Check sheet for the modelled part. Datum: model origin and axes. Units: mm. A direction names the side the tool comes from. Give positions to 0.01 mm unless a question says otherwise; leave off trailing zeros. Loops run counter-clockwise (first coordinate to the right, second up) from the corner with the lowest first, then second, coordinate; pieces in that order, holes last. Notation, with made-up numbers: M -19,-38 L 4,-38 A24 ccw 4,-20 Z; hole C 31,63 d9. An arc over 180 degrees is marked long. Write each question's results on one line, items separated by ' | '. Start each with the question number.
1. Material ranges on line 1 along X through (y, z) = (9.1, 15); line 2 along X through (y, z) = (7.45, 15); line 3 along Z through (x, y) = (-14.5, -0.5), recorded low to high.
2. Draft check along X on faces 6 (the flat face through (4, 11, -25)), 7 (the flat face through (-12.25, 5, -50)), 8 (the flat face through (16, 8, 19)), 9 (the flat face through (20, 4, -26)). Enter one of: pulls with the +X half, pulls with the -X half, needs draft (parallel to the pull), parting line crosses it, or undercut.
3. Sectioned sample at A-A on y = -3.5. Record the cut outline in (x, z).
4. Tool access check on faces 1 (the flat face through (3, 1, -25)), 2 (the flat face through (9, 11, -35.75)), 3 (the flat face through (-12, 8, -65)), 4 (the flat face through (-15, 8, -63)), 5 (the flat face through (7, 14, -39)). Record the directions out of +Z, -Z, +X, -X, +Y, -Y that give a thin tool (end or side, any length) a straight path to the whole face; none if there is none.
5. Go/stop test with flat-tipped pins: pin 1 (1.5 mm diameter, centred on y = 8, z = -26, fed in from -X); pin 2 (12 mm diameter, centred on x = -2.5, y = 6, fed in from -Z); pin 3 (1.5 mm diameter, centred on x = 0.5, z = -25.5, fed in from -Y). Record where each tip stops, or that it passes through.
6. Sectioned sample at C-C on z = -65. Record the cut outline in (x, y).
7. Sectioned sample at B-B on x = -16. Give the number of separate pieces and of enclosed holes in the cut face, and give its area (3 significant figures).
```python
from build123d import *

# Parameters (mm, degrees)
SKETCH1_W                  = 40
SKETCH1_H                  = 22
BOSS_EXTRUDE1_DEPTH        = 11
SKETCH2_W                  = 40
SKETCH2_H                  = 22
SKETCH2_R                  = 7.843750423
BOSS_EXTRUDE2_DEPTH        = 5
SKETCH3_W                  = 24.5
SKETCH3_H                  = 15.5
CUT_EXTRUDE1_DEPTH         = 7.75
FILLET1_R                  = 7.75
SKETCH4_R                  = 5
CUT_EXTRUDE2_DEPTH         = 36.805900352
SKETCH5_W                  = 8
SKETCH5_H                  = 8
SKETCH5_R                  = 1.905800151
BOSS_EXTRUDE3_DEPTH        = 6
CUT_EXTRUDE3_START         = -3
SKETCH6_R                  = 3
SKETCH6_R_2                = 1.905800151
CUT_EXTRUDE3_DEPTH         = 3
SKETCH7_W                  = 16
SKETCH7_H                  = 16.5
BOSS_EXTRUDE5_DEPTH        = 28
MIRROR14_COPY_1_SKETCH_W   = 8
MIRROR14_COPY_1_SKETCH_H   = 8
MIRROR14_COPY_1_SKETCH_R   = 1.905800151
MIRROR14_COPY_1_DEPTH      = 6
MIRROR14_START             = -3
MIRROR14_COPY_2_SKETCH_R   = 3
MIRROR14_COPY_2_SKETCH_R_2 = 1.905800151
MIRROR14_COPY_2_DEPTH      = 3
FILLET1_OF_MIRROR14_R      = 7.75
SKETCH9_W                  = 28
SKETCH9_H                  = 3
BOSS_EXTRUDE6_DEPTH        = 18
CUT_EXTRUDE4_DEPTH         = 10
CUT_EXTRUDE5_DEPTH         = 73.919476136
CUT_EXTRUDE5_DEPTH_BACK    = 73.919476136
SKETCH11_R                 = 1.75
CUT_EXTRUDE6_DEPTH         = 76.121568141
CUT_EXTRUDE6_DEPTH_BACK    = 76.121568141
SKETCH12_R                 = 1.75
CUT_EXTRUDE9_DEPTH         = 12
CUT_EXTRUDE11_START        = -10
SKETCH16_R                 = 4
SKETCH16_R_2               = 1.75
SKETCH16_W                 = 10
SKETCH16_H                 = 6.5
CUT_EXTRUDE11_DEPTH        = 10
FILLET2_R                  = 2
CUT_EXTRUDE12_START        = -3
SKETCH17_R                 = 1.75
CUT_EXTRUDE12_DEPTH        = 3


# Some blends are built 0.0001 mm under size
with BuildPart() as part:
    # Sketch1 → Boss-Extrude1 (new body)
    with BuildSketch(Plane(origin=(0, 0, 0), x_dir=(1, 0, 0), z_dir=(0, 1, 0))):
        Rectangle(SKETCH1_W, SKETCH1_H)
    boss_extrude1 = extrude(amount=BOSS_EXTRUDE1_DEPTH)

    # Sketch2 → Boss-Extrude2 (add)
    with BuildSketch(Plane(origin=(0, 0, 0), x_dir=(1, 0, 0), z_dir=(0, 1, 0))):
        Rectangle(SKETCH2_W, SKETCH2_H)
        with Locations(Location((0, 0, 0), (0, 0, 270))):
            Circle(SKETCH2_R, mode=Mode.SUBTRACT)
    boss_extrude2 = extrude(amount=-BOSS_EXTRUDE2_DEPTH)

    # Sketch3 → Cut-Extrude1 (cut)
    with BuildSketch(Plane(origin=(0, 11, 0), x_dir=(1, 0, 0), z_dir=(0, 1, 0))):
        Rectangle(SKETCH3_W, SKETCH3_H)
    cut_extrude1 = extrude(amount=-CUT_EXTRUDE1_DEPTH, mode=Mode.SUBTRACT)

    # Fillet1
    fillet1_edges = [part.edges().sort_by_distance(p)[0] for p in [
        (0, 3.25, 7.75),
        (0, 3.25, -7.75),
    ]]
    fillet(fillet1_edges, radius=FILLET1_R - 0.0001)  # a hair under: the kernel refuses the full size

    # Sketch4 → Cut-Extrude2 (cut, symmetric)
    with BuildSketch(Plane(origin=(-12.25, 0, 0), x_dir=(0, 0, -1), z_dir=(1, 0, 0))):
        with Locations((0, 11)):
            Circle(SKETCH4_R)
    cut_extrude2 = extrude(amount=CUT_EXTRUDE2_DEPTH, both=True, mode=Mode.SUBTRACT)

    # Sketch5 → Boss-Extrude3 (add)
    with BuildSketch(Plane(origin=(0, 11, 0), x_dir=(1, 0, 0), z_dir=(0, 1, 0))):
        with Locations((16, -15)):
            Rectangle(SKETCH5_W, SKETCH5_H)
        with Locations(Location((16, -15, 0), (0, 0, 270))):
            Circle(SKETCH5_R, mode=Mode.SUBTRACT)
    boss_extrude3 = extrude(amount=-BOSS_EXTRUDE3_DEPTH)

    # Sketch6 → Cut-Extrude3 (cut)
    with BuildSketch(Plane.XZ.offset(-5).offset(CUT_EXTRUDE3_START)):
        with Locations(Location((16, 15, 0), (0, 0, 270))):
            Circle(SKETCH6_R)
        with Locations(Location((16, 15, 0), (0, 0, 90))):
            Circle(SKETCH6_R_2, mode=Mode.SUBTRACT)
    cut_extrude3 = extrude(amount=CUT_EXTRUDE3_DEPTH, mode=Mode.SUBTRACT)

    # Mirror8: Boss-Extrude3, Cut-Extrude3 across plane
    add(boss_extrude3.mirror(Plane(origin=(0, 0, 0), x_dir=(0, 0, 1), z_dir=(1, 0, 0))))
    add(cut_extrude3.mirror(Plane(origin=(0, 0, 0), x_dir=(0, 0, 1), z_dir=(1, 0, 0))), mode=Mode.SUBTRACT)

    # Sketch7 → Boss-Extrude5 (add)
    with BuildSketch(Plane(origin=(0, 0, -11), x_dir=(-1, 0, 0), z_dir=(0, 0, -1))):
        with Locations((-12, 9.25)):
            Rectangle(SKETCH7_W, SKETCH7_H)
    extrude(amount=BOSS_EXTRUDE5_DEPTH)

    # Mirror14: Boss-Extrude1, Boss-Extrude2, Cut-Extrude1, Cut-Extrude2, Boss-Extrude3, Cut-Extrude3 across plane
    add(boss_extrude1.mirror(Plane.XY.offset(-25)))
    add(boss_extrude2.mirror(Plane.XY.offset(-25)))
    add(cut_extrude1.mirror(Plane.XY.offset(-25)), mode=Mode.SUBTRACT)
    add(cut_extrude2.mirror(Plane.XY.offset(-25)), mode=Mode.SUBTRACT)
    add(boss_extrude3.mirror(Plane.XY.offset(-25)))
    add(cut_extrude3.mirror(Plane.XY.offset(-25)), mode=Mode.SUBTRACT)

    # Mirror14 copy 1 sketch → Mirror14 copy 1 (add)
    with BuildSketch(Plane(origin=(0, 11, -50), x_dir=(-1, 0, 0), z_dir=(0, 1, 0))):
        with Locations((16, -15)):
            Rectangle(MIRROR14_COPY_1_SKETCH_W, MIRROR14_COPY_1_SKETCH_H)
        with Locations(Location((16, -15, 0), (0, 0, 270))):
            Circle(MIRROR14_COPY_1_SKETCH_R, mode=Mode.SUBTRACT)
    extrude(amount=-MIRROR14_COPY_1_DEPTH)

    # Mirror14 copy 2 sketch → Mirror14 copy 2 (cut)
    with BuildSketch(Plane(origin=(0, 5, -50), x_dir=(-1, 0, 0), z_dir=(0, -1, 0)).offset(MIRROR14_START)):
        with Locations(Location((16, 15, 0), (0, 0, 270))):
            Circle(MIRROR14_COPY_2_SKETCH_R)
        with Locations(Location((16, 15, 0), (0, 0, 90))):
            Circle(MIRROR14_COPY_2_SKETCH_R_2, mode=Mode.SUBTRACT)
    extrude(amount=MIRROR14_COPY_2_DEPTH, mode=Mode.SUBTRACT)

    # Fillet1 of Mirror14
    fillet1_of_mirror14_edges = [part.edges().sort_by_distance(p)[0] for p in [
        (0, 3.25, -57.75),
        (0, 3.25, -42.25),
    ]]
    fillet(fillet1_of_mirror14_edges, radius=FILLET1_OF_MIRROR14_R - 0.0001)  # a hair under: the kernel refuses the full size

    # Sketch9 → Boss-Extrude6 (add)
    with BuildSketch(Plane.ZY.offset(-4)):
        with Locations((-25, 2.5)):
            Rectangle(SKETCH9_W, SKETCH9_H)
    extrude(amount=BOSS_EXTRUDE6_DEPTH)

    # Sketch10 → Cut-Extrude4 (cut)
    with BuildSketch(Plane(origin=(0, 17.5, 0), x_dir=(1, 0, 0), z_dir=(0, 1, 0))):
        with BuildLine():
            Line((9, 26.25), (9, 23.75))
            Line((9, 23.75), (11.727178029, 23.75))
            ThreePointArc((11.727178029, 23.75), (11.931001031, 24.360286817), (12, 25))
            ThreePointArc((12, 25), (11.931001031, 25.639713183), (11.727178029, 26.25))
            Line((11.727178029, 26.25), (9, 26.25))
        make_face()
        with BuildLine():
            Line((11.727178029, 23.75), (9, 23.75))
            Line((9, 23.75), (9, 26.25))
            Line((9, 26.25), (11.727178029, 26.25))
            ThreePointArc((11.727178029, 26.25), (6, 25), (11.727178029, 23.75))
        make_face()
        with BuildLine():
            ThreePointArc((12, 25), (11.931001031, 24.360286817), (11.727178029, 23.75))
            Line((11.727178029, 23.75), (20, 23.75))
            Line((20, 23.75), (20, 26.25))
            Line((20, 26.25), (11.727178029, 26.25))
            ThreePointArc((11.727178029, 26.25), (11.931001031, 25.639713183), (12, 25))
        make_face()
    extrude(amount=-CUT_EXTRUDE4_DEPTH, mode=Mode.SUBTRACT)

    # Sketch11 → Cut-Extrude5 (cut, two sides: drawn at the far end of the back side and taken through both)
    with BuildSketch(Plane(origin=(0, 7.5, 0), x_dir=(1, 0, 0), z_dir=(0, 1, 0)).offset(-CUT_EXTRUDE5_DEPTH_BACK)):
        with Locations(Location((9, 25, 0), (0, 0, 270))):
            Circle(SKETCH11_R)
    extrude(amount=CUT_EXTRUDE5_DEPTH + CUT_EXTRUDE5_DEPTH_BACK, mode=Mode.SUBTRACT)

    # Sketch12 → Cut-Extrude6 (cut, two sides: drawn at the far end of the back side and taken through both)
    with BuildSketch(Plane.ZY.offset(-4).offset(-CUT_EXTRUDE6_DEPTH_BACK)):
        with Locations((-33, 11)):
            Circle(SKETCH12_R)
    extrude(amount=CUT_EXTRUDE6_DEPTH + CUT_EXTRUDE6_DEPTH_BACK, mode=Mode.SUBTRACT)

    # Sketch15 → Cut-Extrude9 (cut)
    with BuildSketch(Plane(origin=(20, 0, 0), x_dir=(0, 0, -1), z_dir=(1, 0, 0))):
        Polygon((33, 14.175426481), (30.25, 12.58771324), (30.25, 9.41228676), (33, 7.824573519), (35.75, 9.41228676), (35.75, 12.58771324), align=None)
    extrude(amount=-CUT_EXTRUDE9_DEPTH, mode=Mode.SUBTRACT)

    # Sketch16 → Cut-Extrude11 (cut)
    # profile 1 of 2: a face of its own
    with BuildSketch(Plane(origin=(20, 0, 0), x_dir=(0, 0, -1), z_dir=(1, 0, 0)).offset(CUT_EXTRUDE11_START)):
        with Locations((33, 11)):
            Circle(SKETCH16_R)
        with Locations((33, 11)):
            Circle(SKETCH16_R_2, mode=Mode.SUBTRACT)
    # profile 2 of 2: a face of its own
    with BuildSketch(Plane(origin=(20, 0, 0), x_dir=(0, 0, -1), z_dir=(1, 0, 0)).offset(CUT_EXTRUDE11_START)):
        with Locations((34, 14.25)):
            Rectangle(SKETCH16_W, SKETCH16_H)
    extrude(amount=CUT_EXTRUDE11_DEPTH, mode=Mode.SUBTRACT)

    # Chamfer3
    # the kernel refuses this chamfer: 2.5 mm, written as the material it takes off along each edge
    with BuildSketch(Plane(origin=(4.790141486, 11, -37), x_dir=(0, -0.9712202897009368, 0.23818301550116588), z_dir=(1, 0, 0))) as chamfer3_piece_1_section:
        with BuildLine():
            Line((1.641163776, 0), (-0.550057664, 2.010038976))
            Line((-0.550057664, 2.010038976), (-0.598618679, 1.998129825))
            ThreePointArc((-0.598618679, 1.998129825), (-0.296653042, 0.999716345), (-0.048561014, -0.011909151))
            Line((-0.048561014, -0.011909151), (0.011909151, -0.048561014))
            ThreePointArc((0.011909151, -0.048561014), (0.818444442, 0.062835502), (1.633479525, -0.049405994))
            Line((1.633479525, -0.049405994), (1.641163776, 0))
        make_face()
    chamfer3_piece_1 = extrude(amount=20.419717028, mode=Mode.PRIVATE)
    chamfer3_piece_1 = split(chamfer3_piece_1, bisect_by=Plane(origin=(10, 11.063270064, -39.03704072), z_dir=(-1, 0, 0)), keep=Keep.TOP, mode=Mode.PRIVATE)
    chamfer3_piece_1 = split(chamfer3_piece_1, bisect_by=Plane(origin=(7.395070743, 11.063270064, -39), z_dir=(0, 0, -1)), keep=Keep.TOP, mode=Mode.PRIVATE)
    add(chamfer3_piece_1, mode=Mode.SUBTRACT)
    with BuildSketch(Plane(origin=(10, 11, -37), x_dir=(0, -0.9712202897009377, 0.23818301550116178), z_dir=(1, 0, 0))) as chamfer3_piece_2_section:
        with BuildLine():
            Line((1.641163776, 0), (-0.550057664, 2.010038976))
            Line((-0.550057664, 2.010038976), (-0.598618679, 1.998129825))
            ThreePointArc((-0.598618679, 1.998129825), (-0.296653042, 0.999716345), (-0.048561014, -0.011909151))
            Line((-0.048561014, -0.011909151), (0.011909151, -0.048561014))
            ThreePointArc((0.011909151, -0.048561014), (0.818444442, 0.062835502), (1.633479525, -0.049405994))
            Line((1.633479525, -0.049405994), (1.641163776, 0))
        make_face()
    chamfer3_piece_2 = extrude(amount=15.209858514, mode=Mode.PRIVATE)
    chamfer3_piece_2 = split(chamfer3_piece_2, bisect_by=Plane(origin=(17.604929257, 10.514615405, -39), z_dir=(0, 0, 1)), keep=Keep.TOP, mode=Mode.PRIVATE)
    add(chamfer3_piece_2, mode=Mode.SUBTRACT)
    with BuildSketch(Plane(origin=(10, 11, -37), x_dir=(0, -0.9712202897009377, 0.23818301550116178), z_dir=(1, 0, 0))) as chamfer3_piece_3_section:
        with BuildLine():
            Line((1.641163776, 0), (-0.550057664, 2.010038976))
            Line((-0.550057664, 2.010038976), (-0.598618679, 1.998129825))
            ThreePointArc((-0.598618679, 1.998129825), (-0.296653042, 0.999716345), (-0.048561014, -0.011909151))
            Line((-0.048561014, -0.011909151), (0.011909151, -0.048561014))
            ThreePointArc((0.011909151, -0.048561014), (0.818444442, 0.062835502), (1.633479525, -0.049405994))
            Line((1.633479525, -0.049405994), (1.641163776, 0))
        make_face()
    chamfer3_piece_3 = extrude(amount=15.209858514, mode=Mode.PRIVATE)
    chamfer3_piece_3 = split(chamfer3_piece_3, bisect_by=Plane(origin=(17.604929257, 11.063270064, -39), z_dir=(0, 0, -1)), keep=Keep.TOP, mode=Mode.PRIVATE)
    add(chamfer3_piece_3, mode=Mode.SUBTRACT)

    # Fillet2
    fillet2_edges = [part.edges().sort_by_distance(p)[0] for p in [
        (11.727178029, 12.5, -23.75),
        (11.727178029, 12.5, -26.25),
    ]]
    fillet(fillet2_edges, radius=FILLET2_R)

    # Sketch17 → Cut-Extrude12 (cut)
    with BuildSketch(Plane.XZ.offset(-1).offset(CUT_EXTRUDE12_START)):
        Polygon((12.175426481, -25), (10.58771324, -22.25), (7.41228676, -22.25), (5.824573519, -25), (7.41228676, -27.75), (10.58771324, -27.75), align=None)
        with Locations(Location((9, -25, 0), (0, 0, 90))):
            Circle(SKETCH17_R, mode=Mode.SUBTRACT)
    extrude(amount=CUT_EXTRUDE12_DEPTH, mode=Mode.SUBTRACT)


solid = part.part
```
Output values:
1) line 1: -20 to -17.91, -14.09 to -12, 12 to 14.09, 17.91 to 20 | line 2: -20 to -19, -13 to -12, 12 to 13, 19 to 20 | line 3: -61 to -39, -11 to 11
2) face 6: pulls with the -X half | face 7: undercut | face 8: needs draft | face 9: pulls with the +X half
3) outline: M -20,-61 L 20,-61 L 20,-39 L -20,-39 Z; M -20,-11 L 20,-11 L 20,11 L -20,11 Z; hole C 0,-50 d15.69; hole C 0,0 d15.69
4) face 1: +X, -X, -Y | face 2: +X | face 3: -Z, +Y, -Y | face 4: -Y | face 5: -Z, +X, -X, +Y
5) pin 1: x = 4 | pin 2: z = -61 | pin 3: y = 1
6) outline: M -20,5 L -19,5 L -19,8 L -17.91,8 L -17.91,11 L -20,11 Z; M -14.09,8 L -13,8 L -13,5 L -12,5 L -12,11 L -14.09,11 Z; M 12,5 L 13,5 L 13,8 L 14.09,8 L 14.09,11 L 12,11 Z; M 17.91,8 L 19,8 L 19,5 L 20,5 L 20,11 L 17.91,11 Z
7) separate pieces: 4 | enclosed holes: 0 | area: 663 mm2
